For this review, take the finished solid that the model builds, in its own axes (mm). A direction names the side the tool comes from. Round coordinates to 2 decimals unless told otherwise and drop trailing zeros. Loops run counter-clockwise (first coordinate to the right, second up) from the corner with the lowest first, then second, coordinate; pieces in that order, holes last. Notation, with made-up numbers: (21.5, -16) -> (48.5, -16) arc R26 cw to (48.5, 14) -> close; hole circle Ø1 at (-33, -22). An arc over 180 degrees is marked (long way). One line per question, with ' | ' between items. Start each with the question number.
1. Draft analysis for pull direction X (two halves, no side actions). For faces 5 (the face through (-846, 5.4, -351)), 6 (the face through (-788.035, 0.811, -324.339)), 7 (the face through (-872.733, 0.789, -303.668)), state which applies: pulls with the +X half, pulls with the -X half, needs draft (parallel to the pull), parting line crosses it, or undercut.
2. For faces 1 (the face through (-845, 3.06, -343)), 2 (the face through (-865, 3, -337.452)), 3 (the face through (-835, 3.06, -350)), 4 (the face through (-871.535, 3, -325)), list the 3-axis set-ups (+Z, -Z, +X, -X, +Y, -Y) from which the entire face can be reached by the end or side of a thin tool; tool diameter is ignored.
3. Consider section D-D (x = -795.5). Write out the cut boundary in (y, z).
4. Consider section A-A (z = -346.5). Write out the cut boundary in (x, y).
5. Consider section C-C (z = -335). Write out the cut boundary in (x, y).
6. Consider section B-B (x = -863). Write out the cut boundary in (y, z), and give its area (3 significant figures).
7. For pin 1 Ø1 at (y, z) = (3, -341.5) entering from +X; pin 2 Ø1.2 at (y, z) = (2.5, -349.5) entering from +X; pin 3 Ø2.5 at (x, z) = (-836.5, -350) entering from +Y, all flat-tipped, find the tip position at first contact; note any pin that passes through.
8. Wall thickness on line 1 along Z through (x, y) = (-843.5, 2.3); line 2 along X through (y, z) = (3.2, -329.5); line 3 along Y through (x, z) = (-843.5, -312): over which ranges is each line inside the solid? List them lowest first.
```python
from build123d import *

# Parameters (mm, degrees)
SKETCH1_R                    = 1.3
PCB_DEPTH                    = 1.6
NVME_M_KEY_SCREW_HOLES_REACH = 946.451
SKETCH2_R                    = 1
SKETCH3_W                    = 6.78
SKETCH3_H                    = 21.82
NVME_M_KEY_CONNECTOR_DEPTH   = 3.08
SKETCH4_W                    = 5.72
SKETCH4_H                    = 13.26
PCI_E_CONNECTOR_DEPTH        = 2.04
SKETCH5_W                    = 5.2
SKETCH5_H                    = 5
INDUCTANCE_DEPTH             = 3.8
SKETCH6_W                    = 3.08
SKETCH6_H                    = 10
SKETCH6_W_2                  = 6
SKETCH6_H_2                  = 3.08
CAPACITORS_DEPTH             = 1.46


with BuildPart() as part:
    # Sketch1 → pcb (new body)
    with BuildSketch(Plane(origin=(0, 0, 0), x_dir=(1, 0, 0), z_dir=(0, 1, 0))):
        with BuildLine():
            Line((-870.635383482, 358.81294964), (-789.135383482, 358.81294964))
            ThreePointArc((-789.135383482, 358.81294964), (-787.014063138, 357.934269984), (-786.135383482, 355.81294964))
            Line((-786.135383482, 355.81294964), (-786.135383482, 305.81294964))
            ThreePointArc((-786.135383482, 305.81294964), (-787.014063138, 303.691629297), (-789.135383482, 302.81294964))
            Line((-789.135383482, 302.81294964), (-870.635383482, 302.81294964))
            ThreePointArc((-870.635383482, 302.81294964), (-872.756703825, 303.691629297), (-873.635383482, 305.81294964))
            Line((-873.635383482, 305.81294964), (-873.635383482, 355.81294964))
            ThreePointArc((-873.635383482, 355.81294964), (-872.756703825, 357.934269984), (-870.635383482, 358.81294964))
        make_face()
        with Locations(Location((-869.235383482, 355.31294964, 0), (0, 0, 270))):
            Circle(SKETCH1_R, mode=Mode.SUBTRACT)
        with Locations(Location((-869.235383482, 306.31294964, 0), (0, 0, 270))):
            Circle(SKETCH1_R, mode=Mode.SUBTRACT)
        with Locations(Location((-811.135383482, 355.31294964, 0), (0, 0, 270))):
            Circle(SKETCH1_R, mode=Mode.SUBTRACT)
        with Locations(Location((-811.135383482, 306.31294964, 0), (0, 0, 270))):
            Circle(SKETCH1_R, mode=Mode.SUBTRACT)
    extrude(amount=PCB_DEPTH)

    # Sketch2 → NVMe-M-Key screw holes (cut, up to next)
    with BuildSketch(Plane(origin=(0, 1.6, 0), x_dir=(1, 0, 0), z_dir=(0, 1, 0)), mode=Mode.PRIVATE) as nvme_m_key_screw_holes_sk1:
        with Locations(Location((-788.335383482, 325.29294964, 0), (0, 0, 270))):
            Circle(SKETCH2_R)
    nvme_m_key_screw_holes_tool1 = extrude(nvme_m_key_screw_holes_sk1.sketch, amount=-NVME_M_KEY_SCREW_HOLES_REACH, mode=Mode.PRIVATE) & part.part
    # Sketch2 → NVMe-M-Key screw holes (cut, up to next)
    with BuildSketch(Plane(origin=(0, 1.6, 0), x_dir=(1, 0, 0), z_dir=(0, 1, 0)), mode=Mode.PRIVATE) as nvme_m_key_screw_holes_sk2:
        with Locations(Location((-808.295383482, 325.29294964, 0), (0, 0, 270))):
            Circle(SKETCH2_R)
    nvme_m_key_screw_holes_tool2 = extrude(nvme_m_key_screw_holes_sk2.sketch, amount=-NVME_M_KEY_SCREW_HOLES_REACH, mode=Mode.PRIVATE) & part.part
    # Sketch2 → NVMe-M-Key screw holes (cut, up to next)
    with BuildSketch(Plane(origin=(0, 1.6, 0), x_dir=(1, 0, 0), z_dir=(0, 1, 0)), mode=Mode.PRIVATE) as nvme_m_key_screw_holes_sk3:
        with Locations(Location((-826.335383482, 325.29294964, 0), (0, 0, 270))):
            Circle(SKETCH2_R)
    nvme_m_key_screw_holes_tool3 = extrude(nvme_m_key_screw_holes_sk3.sketch, amount=-NVME_M_KEY_SCREW_HOLES_REACH, mode=Mode.PRIVATE) & part.part
    # Sketch2 → NVMe-M-Key screw holes (cut, up to next)
    with BuildSketch(Plane(origin=(0, 1.6, 0), x_dir=(1, 0, 0), z_dir=(0, 1, 0)), mode=Mode.PRIVATE) as nvme_m_key_screw_holes_sk4:
        with Locations(Location((-838.335383482, 325.29294964, 0), (0, 0, 270))):
            Circle(SKETCH2_R)
    nvme_m_key_screw_holes_tool4 = extrude(nvme_m_key_screw_holes_sk4.sketch, amount=-NVME_M_KEY_SCREW_HOLES_REACH, mode=Mode.PRIVATE) & part.part
    add(nvme_m_key_screw_holes_tool1.solids().sort_by_distance((-788.335383, 1.6, -325.29295))[0], mode=Mode.SUBTRACT)
    add(nvme_m_key_screw_holes_tool2.solids().sort_by_distance((-808.295383, 1.6, -325.29295))[0], mode=Mode.SUBTRACT)
    add(nvme_m_key_screw_holes_tool3.solids().sort_by_distance((-826.335383, 1.6, -325.29295))[0], mode=Mode.SUBTRACT)
    add(nvme_m_key_screw_holes_tool4.solids().sort_by_distance((-838.335383, 1.6, -325.29295))[0], mode=Mode.SUBTRACT)

    # Sketch3 → NVMe-M-Key connector (add)
    with BuildSketch(Plane(origin=(0, 1.6, 0), x_dir=(1, 0, 0), z_dir=(0, 1, 0))):
        with Locations((-868.145383482, 325.30294964)):
            Rectangle(SKETCH3_W, SKETCH3_H)
    extrude(amount=NVME_M_KEY_CONNECTOR_DEPTH)

    # Sketch4 → PCI-E connector (add)
    with BuildSketch(Plane(origin=(0, 1.6, 0), x_dir=(1, 0, 0), z_dir=(0, 1, 0))):
        with Locations((-864.975383482, 344.081798362)):
            Rectangle(SKETCH4_W, SKETCH4_H)
    extrude(amount=PCI_E_CONNECTOR_DEPTH)

    # Sketch5 → Inductance (add)
    with BuildSketch(Plane(origin=(0, 1.6, 0), x_dir=(1, 0, 0), z_dir=(0, 1, 0))):
        with Locations((-845.985383482, 351.03294964)):
            Rectangle(SKETCH5_W, SKETCH5_H)
    extrude(amount=INDUCTANCE_DEPTH)

    # Sketch6 → Capacitors (add)
    with BuildSketch(Plane(origin=(0, 1.6, 0), x_dir=(1, 0, 0), z_dir=(0, 1, 0))):
        with Locations((-844.925383482, 342.81294964)):
            Rectangle(SKETCH6_W, SKETCH6_H)
        with Locations((-835.215383482, 350.07294964)):
            Rectangle(SKETCH6_W_2, SKETCH6_H_2)
    extrude(amount=CAPACITORS_DEPTH)


solid = part.part
```
Answer block:
1) face 5: needs draft | face 6: undercut | face 7: pulls with the -X half
2) face 1: +Z, +X, +Y | face 2: +X, -X, +Y | face 3: +Z, -Z, +X, +Y | face 4: +Z, -Z, -X, +Y
3) outline: (0, -358.81) -> (1.6, -358.81) -> (1.6, -302.81) -> (0, -302.81) -> close
4) outline: (-873.64, 0) -> (-786.14, 0) -> (-786.14, 1.6) -> (-843.39, 1.6) -> (-843.39, 3.06) -> (-846.47, 3.06) -> (-846.47, 1.6) -> (-862.12, 1.6) -> (-862.12, 3.64) -> (-867.84, 3.64) -> (-867.84, 1.6) -> (-873.64, 1.6) -> close
5) outline: (-873.64, 0) -> (-786.14, 0) -> (-786.14, 1.6) -> (-864.76, 1.6) -> (-864.76, 4.68) -> (-871.54, 4.68) -> (-871.54, 1.6) -> (-873.64, 1.6) -> close
6) outline: (0, -358.81) -> (1.6, -358.81) -> (1.6, -350.71) -> (3.64, -350.71) -> (3.64, -337.45) -> (1.6, -337.45) -> (1.6, -302.81) -> (0, -302.81) -> close | area: 117 mm2
7) pin 1: stops at x = -843.39 | pin 2: stops at x = -832.22 | pin 3: stops at y = 3.06
8) line 1: z = -353.53 to -348.53, -347.81 to -337.81 | line 2: x = -871.54 to -864.76 | line 3: y = 0 to 1.6
